Geometry check sheet. Reference: drawing and pictorial views, mm from the part's lowest x, y, z. Round coordinates to 2 decimals unless told otherwise and drop trailing zeros. Loops run counter-clockwise (first coordinate to the right, second up) from the corner with the lowest first, then second, coordinate; pieces in that order, holes last. Notation, with made-up numbers: M -38,61.5 L -18,61.5 A25 cw -18,84.5 Z; hole C 79.25,-34.75 d9. An arc over 180 degrees is marked long. One line per question, with ' | ' between items. Start each with the question number.
(1) Thickness scan on probe 1 along Y at (x, z) = (45, 4.7); probe 2 along X at (y, z) = (37, 5.65); probe 3 along Y at (x, z) = (7, 2.1). Record the ranges inside material, lowest first. Write a range as [from, to].
(2) Section check A-A (x = 5). Record the boundary of the cut face in (y, z).
(3) Section check C-C (y = 5). Record the boundary of the cut face in (x, z).
(4) Go/stop test with flat-tipped pins: P1, Ø2, axis at x = 36, z = 3, coming from the -Y side; P2, Ø2.5, axis at x = 45, y = 5, coming from the -Z side. Record where each tip stops, or that it passes through.
(5) Section check B-B (z = 1.15). Record the boundary of the cut face in (x, y), and give its area (3 significant figures).
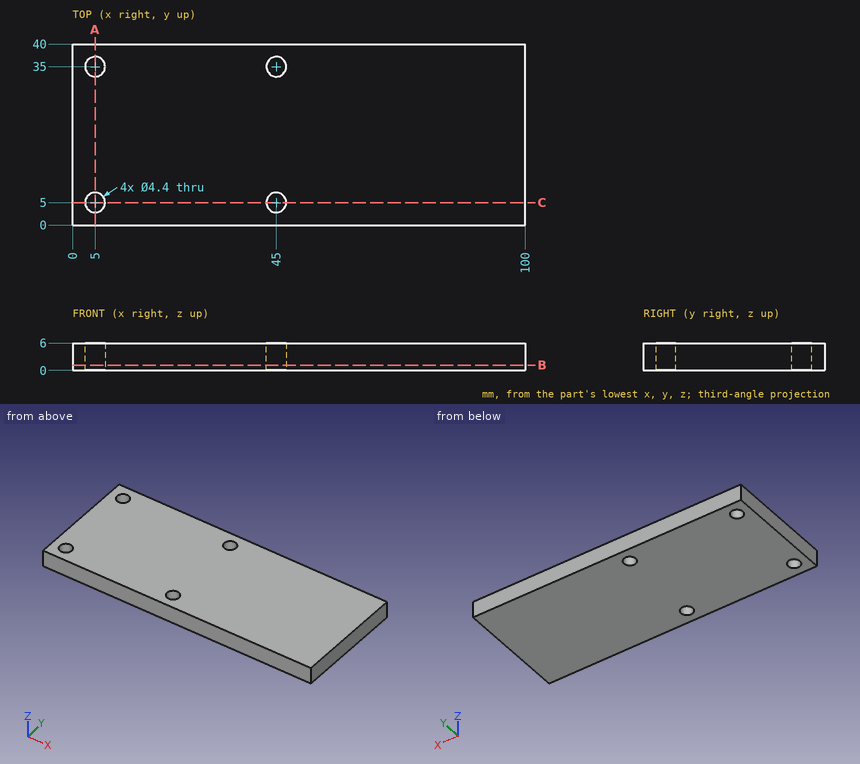
The answers:
1) probe 1: [0, 2.8], [7.2, 32.8], [37.2, 40] | probe 2: [0, 4.08], [5.92, 44.08], [45.92, 100] | probe 3: [0, 4.08], [5.92, 34.08], [35.92, 40]
2) outline: M 0,0 L 2.8,0 L 2.8,6 L 0,6 Z; M 7.2,0 L 32.8,0 L 32.8,6 L 7.2,6 Z; M 37.2,0 L 40,0 L 40,6 L 37.2,6 Z
3) outline: M 0,0 L 2.8,0 L 2.8,6 L 0,6 Z; M 7.2,0 L 42.8,0 L 42.8,6 L 7.2,6 Z; M 47.2,0 L 100,0 L 100,6 L 47.2,6 Z
4) P1: y = 0 | P2: through
5) outline: M 0,0 L 100,0 L 100,40 L 0,40 Z; hole C 5,5 d4.4; hole C 5,35 d4.4; hole C 45,5 d4.4; hole C 45,35 d4.4 | area: 3,940 mm²
